```python
from build123d import *

# Parameters (mm, degrees)
BOSS_EXTRUDE1_DEPTH = 6.2
CUT_EXTRUDE1_REACH  = 42.021
SKETCH2_R           = 1.5


with BuildPart() as part:
    # Sketch1 → Boss-Extrude1 (new body)
    with BuildSketch(Plane(origin=(0, 0, 0), x_dir=(1, 0, 0), z_dir=(0, 1, 0))):
        Polygon((-21, 27.5), (-16, 27.5), (-16, 33.5), (-8, 33.5), (-8, 27.5), (-2.5, 27.5), (-2.5, 21.5), (-4, 21.5), (-4, 17.5), (4, 17.5), (4, 21.5), (2.5, 21.5), (2.5, 27.5), (8, 27.5), (8, 33.5), (16, 33.5), (16, 27.5), (21, 27.5), (21, -27.5), (16, -27.5), (16, -33.5), (8, -33.5), (8, -27.5), (2.5, -27.5), (2.5, -21.5), (4, -21.5), (4, -17.5), (-4, -17.5), (-4, -21.5), (-2.5, -21.5), (-2.5, -27.5), (-8, -27.5), (-8, -33.5), (-16, -33.5), (-16, -27.5), (-21, -27.5), align=None)
    extrude(amount=BOSS_EXTRUDE1_DEPTH)

    # Sketch2 → Cut-Extrude1 (cut, up to next)
    with BuildSketch(Plane(origin=(0, 6.2, 0), x_dir=(1, 0, 0), z_dir=(0, 1, 0)), mode=Mode.PRIVATE) as cut_extrude1_sk1:
        with Locations(Location((15.5, -15.5, 0), (0, 0, 270))):
            Circle(SKETCH2_R)
    cut_extrude1_tool1 = extrude(cut_extrude1_sk1.sketch, amount=-CUT_EXTRUDE1_REACH, mode=Mode.PRIVATE) & part.part
    # Sketch2 → Cut-Extrude1 (cut, up to next)
    with BuildSketch(Plane(origin=(0, 6.2, 0), x_dir=(1, 0, 0), z_dir=(0, 1, 0)), mode=Mode.PRIVATE) as cut_extrude1_sk2:
        with Locations(Location((-15.5, -15.5, 0), (0, 0, 270))):
            Circle(SKETCH2_R)
    cut_extrude1_tool2 = extrude(cut_extrude1_sk2.sketch, amount=-CUT_EXTRUDE1_REACH, mode=Mode.PRIVATE) & part.part
    # Sketch2 → Cut-Extrude1 (cut, up to next)
    with BuildSketch(Plane(origin=(0, 6.2, 0), x_dir=(1, 0, 0), z_dir=(0, 1, 0)), mode=Mode.PRIVATE) as cut_extrude1_sk3:
        with Locations(Location((-15.5, 15.5, 0), (0, 0, 270))):
            Circle(SKETCH2_R)
    cut_extrude1_tool3 = extrude(cut_extrude1_sk3.sketch, amount=-CUT_EXTRUDE1_REACH, mode=Mode.PRIVATE) & part.part
    # Sketch2 → Cut-Extrude1 (cut, up to next)
    with BuildSketch(Plane(origin=(0, 6.2, 0), x_dir=(1, 0, 0), z_dir=(0, 1, 0)), mode=Mode.PRIVATE) as cut_extrude1_sk4:
        with Locations(Location((15.5, 15.5, 0), (0, 0, 270))):
            Circle(SKETCH2_R)
    cut_extrude1_tool4 = extrude(cut_extrude1_sk4.sketch, amount=-CUT_EXTRUDE1_REACH, mode=Mode.PRIVATE) & part.part
    add(cut_extrude1_tool1.solids().sort_by_distance((15.5, 6.2, 15.5))[0], mode=Mode.SUBTRACT)
    add(cut_extrude1_tool2.solids().sort_by_distance((-15.5, 6.2, 15.5))[0], mode=Mode.SUBTRACT)
    add(cut_extrude1_tool3.solids().sort_by_distance((-15.5, 6.2, -15.5))[0], mode=Mode.SUBTRACT)
    add(cut_extrude1_tool4.solids().sort_by_distance((15.5, 6.2, -15.5))[0], mode=Mode.SUBTRACT)


solid = part.part
```
Input: part model. Units: mm. Frame: model coordinates. A direction names the side the tool comes from. Coordinates: 2 decimals unless noted, no trailing zeros. Write each loop counter-clockwise with the first axis right and the second up, starting at its lowest first coordinate (ties: lowest second). Pieces come first, ordered by that corner, then holes. Notation, with made-up numbers: (53.25, -34) -> (69.25, -34) arc R18 cw to (69.25, -25) -> close; hole circle Ø10 at (-27.75, 34). An arc over 180 degrees is marked (long way). Write each question's results on one line, items separated by ' | '.
Item 1: Mould query, pull axis X, two halves, no side actions, for faces 4 (the flat face through (0, 3, -17.5)), 5 (the flat face through (-5, 3, 27.5)), 6 (the flat face through (16, 3, 30)), 7 (the flat face through (12, 3, 33.5)). Classes: +X half, -X half, draft (parallel to the pull), parting line (faces both ways), or undercut.
Conclusion:
face 4: undercut | face 5: undercut | face 6: +X half | face 7: draft
Item 2: Material intervals for probe 1 along X at (y, z) = (4.25, -15.5); probe 2 along X at (y, z) = (3.25, 23); probe 3 along Z at (x, y) = (14.5, 4.75), sorted ascending.
Conclusion:
probe 1: x = -21 to -17, -14 to 14, 17 to 21 | probe 2: x = -21 to -2.5, 2.5 to 21 | probe 3: z = -33.5 to -16.62, -14.38 to 14.38, 16.62 to 33.5
Item 3: Set-up query: faces 1 (the flat face through (-8, 3, -31)), 2 (the flat face through (-2.5, 3, 24)), 3 (the flat face through (3, 3, -21.5)). Return all of +Z, -Z, +X, -X, +Y, -Y with unobstructed straight access to the full face (end or side cutting, diameter ignored); none if empty.
Conclusion:
face 1: -Z, +Y, -Y | face 2: +Z, +Y, -Y | face 3: +Y, -Y
Item 4: Section query D-D on x = 7. Return loops of the section in (y, z), plus the area to 3 significant figures.
Conclusion:
outline: (0, -27.5) -> (6.2, -27.5) -> (6.2, 27.5) -> (0, 27.5) -> close | area: 341 mm^2
Item 5: Section query C-C on y = 4.5. Count the separate pieces of the cut face and the enclosed holes in it, plus the area to 3 significant figures.
Conclusion:
separate pieces: 1 | enclosed holes: 4 | area: 2,350 mm^2
Item 6: Pin query (flat end, axial travel): pin 1 Ø1.5 at (x, y) = (5, 2.5) entering from -Z; pin 2 Ø1.9 at (x, y) = (1, 3) entering from -Z; pin 3 Ø3 at (y, z) = (4, 31.5) entering from +X. Return the tip coordinate at first contact, or that it passes through.
Conclusion:
pin 1: stops at z = -27.5 | pin 2: stops at z = -17.5 | pin 3: stops at x = 16
Item 7: Section query B-B on z = -15.5. Return loops of the section in (x, y).
Conclusion:
outline: (-21, 0) -> (-17, 0) -> (-17, 6.2) -> (-21, 6.2) -> close; (-14, 0) -> (14, 0) -> (14, 6.2) -> (-14, 6.2) -> close; (17, 0) -> (21, 0) -> (21, 6.2) -> (17, 6.2) -> close
Item 8: Section query A-A on z = -24. Return loops of the section in (x, y), plus the area to 3 significant figures.
Conclusion:
outline: (-21, 0) -> (-2.5, 0) -> (-2.5, 6.2) -> (-21, 6.2) -> close; (2.5, 0) -> (21, 0) -> (21, 6.2) -> (2.5, 6.2) -> close | area: 229 mm^2
